Read the model definition and answer for the solid it produces. Units are mm, in the model's axes. Give positions to 0.01 mm unless a question says otherwise; leave off trailing zeros. Order: outer loops, then holes, each group sorted by start corner. A loop starts at its lowest first (then second) coordinate and runs counter-clockwise, first axis right, second up. Notation, with made-up numbers: (-28.75, -5) - (5.25, -5) arc R16 cw to (5.25, 18) - close; hole circle Ø8 at (-11.5, -17). An arc over 180 degrees is marked (long way). Return JSON: item names as keys, results as strings.
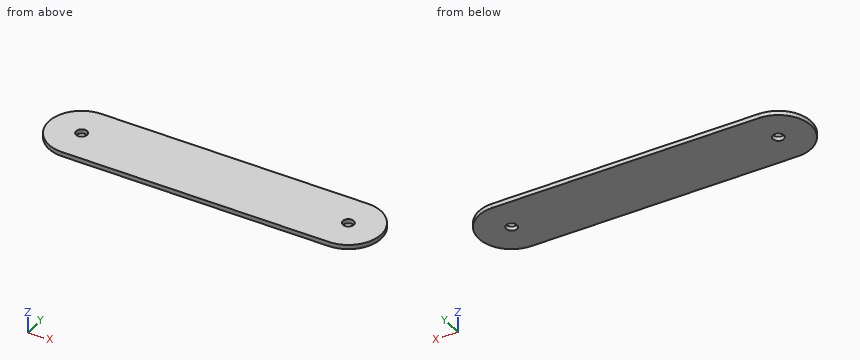
Autodesk Inventor part; units mm, degrees
ref_plane "YZ Plane" through (0, 0, 0) normal (1, 0, 0) x (0, 1, 0)
ref_plane "XZ Plane" through (0, 0, 0) normal (0, 1, 0) x (-1, 0, 0)
ref_plane "XY Plane" through (0, 0, 0) normal (0, 0, 1) x (1, 0, 0)
sketch "Sketch1" plane through (0, 0, 0) normal (0, 0, 1) x (1, 0, 0)
  line L0 (-60, 0) -> (60, 0) construction
  line L1 (-60, -15) -> (60, -15)
  line L2 (60, 15) -> (-60, 15)
  arc A0 (-60, 15) -> (-60, -15) centre (-60, 0) ccw
  arc A1 (60, -15) -> (60, 15) centre (60, 0) ccw
  circle A2 centre (-60, 0) radius 2.5
  circle A3 centre (60, 0) radius 2.5
  line L3 (0, 15) -> (0, -15) construction
  point P0 (0, 0)
  point P1 (0, 0)
  point P2 (0, 0)
  point P3 (0, 0)
  dimension "d37" = 120
  dimension "d38" = 15
  dimension "d39" = 120
  dimension "d40" = 5
extrude "Plate1" add sketch "Sketch1" against normal blind 2
equation "\"d15\" = Thickness"
equation "\"BendRadius\" = Thickness"
equation "\"BendReliefWidth\" = Thickness"
equation "\"BendReliefDepth\" = 0.5 * Thickness"
equation "\"CornerReliefSize\" = 4 * Thickness"
equation "\"MinimumRemnant\" = 2 * Thickness"
equation "\"TransitionRadius\" = BendRadius"
equation "\"JacobiRadiusSize\" = BendRadius"
equation "\"GapSize\" = Thickness"
properties part number "ДМФ 01 15 Барабан усилитель борта"
Q1. A cutting plane is placed at C-C (y = -10.75). Write down the section's boundary in (x, z).
Values:
{"outline": "(-70.46, -2) - (70.46, -2) - (70.46, 0) - (-70.46, 0) - close"}
Q2. A cutting plane is placed at A-A (y = 0). Write down the section's boundary in (x, z).
Values:
{"outline": "(-75, -2) - (-62.5, -2) - (-62.5, 0) - (-75, 0) - close; (-57.5, -2) - (57.5, -2) - (57.5, 0) - (-57.5, 0) - close; (62.5, -2) - (75, -2) - (75, 0) - (62.5, 0) - close"}
Q3. Given pin 1 (4 mm diameter, centred on x = -60, y = 0, fed in from +Z), flat-ended and moving along its own axis, determine where the tip first touches the part or whether it passes through.
Values:
{"pin 1": "passes through"}
Q4. A cutting plane is placed at B-B (z = -0.9). Write down the section's boundary in (x, y), and give its area (3 significant figures).
Values:
{"outline": "(-60, -15) - (60, -15) arc R15 ccw to (60, 15) - (-60, 15) arc R15 ccw to start; hole circle Ø5 at (-60, 0); hole circle Ø5 at (60, 0)", "area": "4,270 mm²"}
Q5. Consider L1, parallel to Y at x = 60, z = -1.2; L2, parallel to X at y = 0.5, z = -1.7; L3, parallel to X at y = 12.5, z = -1.5. Determine where each line is inside the solid, lowest interval first.
Values:
{"L1": "y = -15 to -2.5, 2.5 to 15", "L2": "x = -74.99 to -62.45, -57.55 to 57.55, 62.45 to 74.99", "L3": "x = -68.29 to 68.29"}
